Work out the finished part from the listing and answer in its coordinate system (mm). Face numbers are marked on the shaded views. Round coordinates to 2 decimals unless told otherwise and drop trailing zeros. Write each loop counter-clockwise with the first axis right and the second up, starting at its lowest first coordinate (ties: lowest second). Pieces come first, ordered by that corner, then holes.
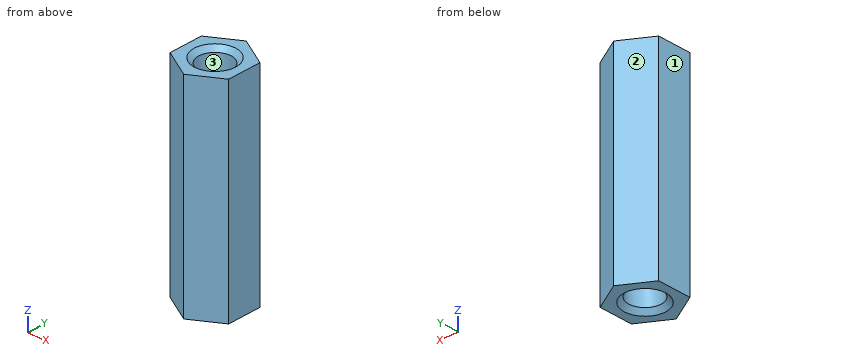
Autodesk Inventor part; units mm, degrees
ref_plane "YZ Plane" through (0, 0, 0) normal (1, 0, 0) x (0, 1, 0)
ref_plane "XZ Plane" through (0, 0, 0) normal (0, 1, 0) x (-1, 0, 0)
ref_plane "XY Plane" through (0, 0, 0) normal (0, 0, 1) x (1, 0, 0)
sketch "Sketch1" plane through (0, 0, 0) normal (0, 0, 1) x (1, 0, 0)
  circle A0 centre (0, 0) radius 7.255
  line L0 (0, -7.255) -> (-6.283, -3.6275)
  line L1 (-6.283, -3.6275) -> (-6.283, 3.6275)
  line L2 (-6.283, 3.6275) -> (0, 7.255)
  line L3 (0, 7.255) -> (6.283, 3.6275)
  line L4 (6.283, 3.6275) -> (6.283, -3.6275)
  line L5 (6.283, -3.6275) -> (0, -7.255)
  dimension "d0" = 14.51
extrude "Extrusion1" add sketch "Sketch1" along normal mid plane 44.28 contours L4 L5 L0 L1 L2 L3
sketch "Sketch2" plane through (0, 0, 22.14) normal (0, 0, 1) x (1, 0, 0)
  circle A0 centre (0, 0) radius 4.3621
hole "Hole1" at (0, 0, 22.14) direction (0, 0, -1) diameter 6.9088 end through all
chamfer "Chamfer1" distance 1 angle 45 1 edges at (0, 3.4544, 22.14)
chamfer "Chamfer2" distance 1 angle 45 1 edges at (0, 3.4544, -22.14)
properties part number "CNC- Hexagonal Bit"
Q1. The mould has two halves that part along Y. Classify the marked faces 1, 2 and 3: +Y half, -Y half, draft (parallel to the pull), parting line (faces both ways), or undercut.
Q2. Find the intervals of material crossed by L1, parallel to X at y = 0, z = -7; L2, parallel to Y at x = 0, z = 4.5 (3 decimals); L3, parallel to X at y = 0.75, z = 11, in increasing order.
Q3. Given pin 1 (3 mm diameter, centred on x = -3.5, z = -14, fed in from -Y); pin 2 (2 mm diameter, centred on x = 3.5, y = -2, fed in from +Z); pin 3 (1.5 mm diameter, centred on x = -3.5, z = -13, fed in from +Y); pin 4 (1 mm diameter, centred on x = -4.5, z = 2, fed in from +Y), each flat-ended and moving along its own axis, determine where each tip first touches the part or whether it passes through.
Q4. Find section A-A (y = 0). Determine the outline of the cut face in (x, z), plus the area to 3 significant figures.
Q5. Find section B-B (z = 5). Determine the outline of the cut face in (x, y) (1 decimal).
Q6. Find section C-C (y = -5.75). Determine the outline of the cut face in (x, z), plus the area to 3 significant figures.
Report:
1. face 1: draft
1. face 2: +Y half
1. face 3: undercut
2. L1: x = -6.28 to -3.45, 3.45 to 6.28
2. L2: y = -7.255 to -3.454, 3.454 to 7.255
2. L3: x = -6.28 to -3.37, 3.37 to 6.28
3. pin 1: stops at y = -6.1
3. pin 2: stops at z = 22.14
3. pin 3: stops at y = 5.67
3. pin 4: stops at y = 4.95
4. outline: (-6.28, -22.14) - (-4.45, -22.14) - (-3.45, -21.14) - (-3.45, 21.14) - (-4.45, 22.14) - (-6.28, 22.14) - close; (3.45, -21.14) - (4.45, -22.14) - (6.28, -22.14) - (6.28, 22.14) - (4.45, 22.14) - (3.45, 21.14) - close
4. area: 249 mm2
5. outline: (-6.3, -3.6) - (0, -7.3) - (6.3, -3.6) - (6.3, 3.6) - (0, 7.3) - (-6.3, 3.6) - close; hole circle Ø6.9 at (0, 0)
6. outline: (-2.61, -22.14) - (2.61, -22.14) - (2.61, 22.14) - (-2.61, 22.14) - close
6. area: 231 mm2
